Design review of the part built by this model. Coordinates are the model's own, in mm. Give positions to 0.01 mm unless a question says otherwise; leave off trailing zeros. Answer in a Markdown table with one row per item. Add a question column.
(1) Consider section A-A on z = 1.75. Count the separate pieces of the cut face and the enclosed holes in it, then the cut area to 3 significant figures.
(2) For pin 1 (8 mm diameter, centred on x = 37.33, y = 136.25, fed in from +Z), flat-tipped, find the tip position at first contact; note if it passes through.
(3) For line 1 (Y direction, x = 86, z = 3.75), list the stretches that pass through material, from the lowest coordinate up.
from build123d import *

# Parameters (mm, degrees)
SKETCH1_W                   = 250
SKETCH1_H                   = 250
BOSS_EXTRUDE1_DEPTH         = 6.35
FILLET1_R                   = 10
TAP_DRILL_FOR_M6X1_0_TAP1_D = 5
TAP_DRILL_FOR_M6X1_0_TAP2_D = 5
TAP_DRILL_FOR_M6X1_0_TAP3_D = 5


with BuildPart() as part:
    # Sketch1 → Boss-Extrude1 (new body)
    with BuildSketch(Plane(origin=(-15.018309821, 0, 0), x_dir=(1, 0, 0), z_dir=(0, 0, 1))):
        with Locations((75.170478225, 83.366123253)):
            Rectangle(SKETCH1_W, SKETCH1_H)
    extrude(amount=BOSS_EXTRUDE1_DEPTH)

    # Fillet1
    fillet1_edges = [part.edges().sort_by_distance(p)[0] for p in [
        (-64.847831597, 208.366123253, 3.175),
        (185.152168403, 208.366123253, 3.175),
        (185.152168403, -41.633876747, 3.175),
        (-64.847831597, -41.633876747, 3.175),
    ]]
    fillet(fillet1_edges, radius=FILLET1_R)

    # Tap Drill for M6x1.0 Tap1 (through all)
    with Locations(Plane.XY.offset(6.35)):
        with Locations((37.327836752, 136.24557957), (88.127836752, 136.24557957), (37.3593105, 124.457685542), (88.127838497, 126.24557957)):
            Hole(TAP_DRILL_FOR_M6X1_0_TAP1_D / 2)

    # Tap Drill for M6x1.0 Tap2 (through all)
    with Locations(Plane.XY.offset(6.35)):
        with Locations((120.892593903, 187.375248984), (171.692593903, 187.375248984), (171.692593906, 177.375248984), (120.892593906, 177.375248984), (-48.228620318, 187.375248984), (2.571379682, 187.375248984), (2.571379686, 177.375248984), (-48.228620318, 177.375248984), (-48.228620318, 64.020452142), (-48.228620318, 54.020452142), (2.571379682, 64.020452142), (2.571379682, 54.020452142), (2.571379682, 4.309579467), (2.571379682, -5.690420533), (-48.228620318, 4.309579467), (-48.228620318, -5.690420533), (120.892593903, 64.020452142), (171.692593903, 64.020452142), (171.692593903, 54.020452142), (120.892593903, 54.020452142), (120.892593903, 4.309579467), (171.692593903, 4.309579467), (171.692593903, -5.690420533), (120.892593903, -5.690420533), (-48.228620318, 136.245579568), (-48.228620318, 126.245579568), (2.571379686, 136.245579568), (2.571379686, 126.245579568), (120.892593906, 136.245579568), (120.892593906, 126.245579568), (171.692593906, 136.245579568), (171.692593906, 126.245579568)):
            Hole(TAP_DRILL_FOR_M6X1_0_TAP2_D / 2)

    # Tap Drill for M6x1.0 Tap3 (through all)
    with Locations(Plane.XY.offset(6.35)):
        with Locations((38.064970254, 187.375245165), (88.864970254, 187.37524898), (88.875056728, 177.375254067), (38.075056728, 177.375250252), (36.642065603, 64.020452168), (87.442065603, 64.02045214), (87.436525124, 54.020453675), (36.636525124, 54.020453703), (39.131440217, 4.309560284), (89.931440217, 4.30957947), (89.954059606, -5.690394948), (39.154059606, -5.690414135)):
            Hole(TAP_DRILL_FOR_M6X1_0_TAP3_D / 2)


solid = part.part
Values follow:
| question | item | result |
|---|---|---|
| 1 | separate pieces | 1 |
| 1 | enclosed holes | 48 |
| 1 | area | 61,500 mm2 |
| 2 | pin 1 | z = 6.35 |
| 3 | line 1 | -41.63 to 51.97, 56.07 to 61.98, 66.06 to 124.93, 127.56 to 134.93, 137.56 to 208.37 |
